```python
from build123d import *

# Parameters (mm, degrees)
F0_R     = 9.525
F1_DEPTH = 25.4
F3_DEPTH = 25.401
F4_DEPTH = 11.1252
F6_DEPTH = 9.525
F7_R     = 0.762
F8_R     = 0.762
F9_R     = 0.762


with BuildPart() as f1:
    # F0 (on Front) → F1 (new body)
    with BuildSketch(Plane.XZ):
        Circle(F0_R)
    extrude(amount=F1_DEPTH)

    # F2 (on Front) → F3 (cut, through all)
    with BuildSketch(Plane.XZ):
        with BuildLine():
            ThreePointArc((4.7625, 0), (3.367596, 3.367596), (0, 4.7625))
            ThreePointArc((0, 4.7625), (-3.367596, 3.367596), (-4.7625, 0))
            ThreePointArc((-4.7625, 0), (-3.367596, -3.367596), (0, -4.7625))
            ThreePointArc((0, -4.7625), (3.367596, -3.367596), (4.7625, 0))
        make_face()
    extrude(amount=F3_DEPTH, mode=Mode.SUBTRACT)

    # F2 (on Front) → F4 (cut)
    with BuildSketch(Plane.XZ):
        with BuildLine():
            Line((0, 4.7625), (-4.7625, 4.7625))
            Line((-4.7625, 4.7625), (-4.7625, 0))
            ThreePointArc((-4.7625, 0), (-3.367596, 3.367596), (0, 4.7625))
        make_face()
        with BuildLine():
            Line((4.7625, 4.7625), (0, 4.7625))
            ThreePointArc((0, 4.7625), (3.367596, 3.367596), (4.7625, 0))
            Line((4.7625, 0), (4.7625, 4.7625))
        make_face()
        with BuildLine():
            ThreePointArc((0, -4.7625), (-3.367596, -3.367596), (-4.7625, 0))
            Line((-4.7625, 0), (-4.7625, -4.7625))
            Line((-4.7625, -4.7625), (0, -4.7625))
        make_face()
        with BuildLine():
            Line((4.7625, -4.7625), (4.7625, 0))
            ThreePointArc((4.7625, 0), (3.367596, -3.367596), (0, -4.7625))
            Line((0, -4.7625), (4.7625, -4.7625))
        make_face()
    extrude(amount=F4_DEPTH, mode=Mode.SUBTRACT)

    # F5 (on face) → F6 (cut)
    with BuildSketch(Plane.XZ.offset(25.4)):
        Polygon((3.65125, 6.324151), (-3.65125, 6.324151), (-7.3025, 0), (-3.65125, -6.324151), (3.65125, -6.324151), (7.3025, 0), align=None)
    extrude(amount=-F6_DEPTH, mode=Mode.SUBTRACT)

    # F7
    f7_edges = [f1.edges().sort_by_distance(p)[0] for p in [
        (-9.525, 0, 0),
        (-9.525, -25.4, 0),
    ]]
    fillet(f7_edges, radius=F7_R)

    # F8
    f8_edges = [f1.edges().sort_by_distance(p)[0] for p in [
        (3.65125, -20.6375, 6.324151),
        (3.65125, -20.6375, -6.324151),
        (-3.65125, -20.6375, -6.324151),
        (-7.3025, -20.6375, 0),
        (-3.65125, -20.6375, 6.324151),
        (7.3025, -20.6375, 0),
    ]]
    fillet(f8_edges, radius=F8_R)

    # F9
    f9_edges = [f1.edges().sort_by_distance(p)[0] for p in [
        (0, -15.875, 6.324151),
    ]]
    fillet(f9_edges, radius=F9_R)


solid = f1.part
```
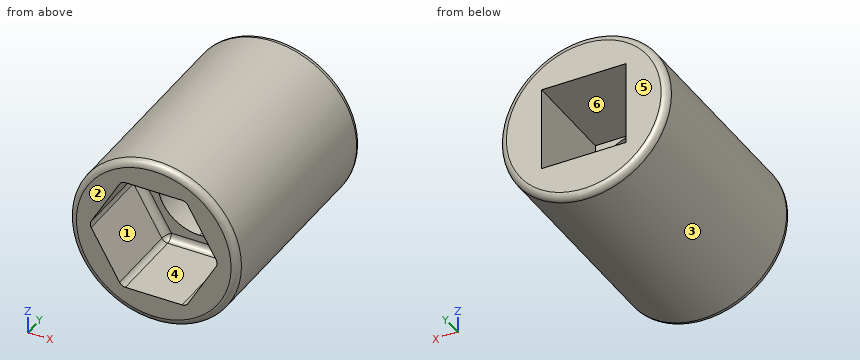
Here's how the part is built. I have some questions about the finished solid (model axes, mm). Face numbers are marked on the shaded views. A direction names the side the tool comes from. Give positions to 0.01 mm unless a question says otherwise; leave off trailing zeros. Loops run counter-clockwise (first coordinate to the right, second up) from the corner with the lowest first, then second, coordinate; pieces in that order, holes last. Notation, with made-up numbers: (-12.5, 89) -> (21.5, 89) arc R16 ccw to (21.5, 112) -> close; hole circle Ø7 at (-32.75, -24). An arc over 180 degrees is marked (long way). Use one line per item in the form item = value. Start each with the question number.
1) Thinking about a two-plate mould opening in X: for the marked faces 1, 2, 3 and 4, which applies, +X half, -X half, draft (parallel to the pull), parting line (faces both ways), or undercut?
2) Which directions (+Z, -Z, +X, -X, +Y, -Y) give clear straight access to the entire face, cutting with the end or side of a thin tool? Please do the marked faces 5 and 6.
3) For P1, Ø4, axis at x = -2, z = 2, coming from the +Y side; P2, Ø4, axis at y = -12, z = 6.5, coming from the +X side (3 decimals); P3, Ø8, axis at y = -3, z = 6, coming from the -X side, each with a flat end and sliding along its axis, tell me the tip position at first contact or that it passes through.
4) Please list where these lines run through material, in increasing order: line 1 along Z through (x, y) = (-6.25, -0.75); line 2 along Z through (x, y) = (-2.5, -13.5); line 3 along X through (y, z) = (-15, 3.5).
5) Imagine slicing it at A-A (y = -17.25). Please give me the cut outline in (x, z) (3 decimals).
Check values:
q1.face_1 = undercut
q1.face_2 = draft
q1.face_3 = parting line
q1.face_4 = undercut
q2.face_5 = +Z, -Z, +X, -X, +Y
q2.face_6 = +Y
q3.P1 = -11.13
q3.P2 = 8.395
q3.P3 = -9.31
q4.line_1 = -7.19 to 7.19
q4.line_2 = -9.19 to -4.05, 4.05 to 9.19
q4.line_3 = -8.86 to -3.23, 3.23 to 8.86
q5.outline = circle Ø19.05 at (0, 0); hole (-7.083, -0.381) -> (-3.871, -5.943) arc R0.762 ccw to (-3.211, -6.324) -> (3.211, -6.324) arc R0.762 ccw to (3.871, -5.943) -> (7.083, -0.381) arc R0.762 ccw to (7.083, 0.381) -> (3.871, 5.943) arc R0.762 ccw to (3.211, 6.324) -> (-3.211, 6.324) arc R0.762 ccw to (-3.871, 5.943) -> (-7.083, 0.381) arc R0.762 ccw to start
